The model under review builds one solid part; all positions refer to its coordinate system, in mm. Coordinates: 2 decimals unless noted, no trailing zeros. Order: outer loops, then holes, each group sorted by start corner. A loop starts at its lowest first (then second) coordinate and runs counter-clockwise, first axis right, second up. Notation, with made-up numbers: M 55,29 L 61,29 A23 cw 61,49 Z; hole C -3,19 d5. An arc over 180 degrees is marked long. Answer as CSV lines item,"result". Start each with the question number.
Q1. The part is to be moulded in two halves that separate along Z. For faces 1 (the face through (-3.45, -1.503, -19.963)), 2 (the face through (60.5, -2, -7)), 3 (the face through (45.473, -1.503, -11.382)), say which applies: +Z half, -Z half, draft (parallel to the pull), parting line (faces both ways), or undercut.
Q2. For P1, Ø6, axis at x = -46, z = 3, coming from the +Y side; P2, Ø1.5, axis at x = -42.5, y = -1.5, coming from the +Z side, all flat-tipped, find the tip position at first contact; note any pin that passes through.
Q3. Consider section A-A on x = -41. Write out the cut boundary in (y, z), and give its area (3 significant figures).
Q4. Consider section C-C on y = -0.8. Write out the cut boundary in (x, z).
Q5. Consider section D-D on x = -18. Write out the cut boundary in (y, z).
Q6. Wall thickness on L1, parallel to X at y = -0.15, z = -12; L2, parallel to X at y = -0.75, z = -11.5; L3, parallel to X at y = -2.5, z = 10.5: over which ranges is each line inside the solid? List them lowest first. Write a range as [from, to].
Q7. Consider section B-B on z = 5. Write out the cut boundary in (x, y).
from build123d import *

# Parameters (mm, degrees)
F0_R     = 2.7500072
F1_DEPTH = 3.048


# Not quite as in the source:
# - ends of sketch curves that miss each other by under 0.0002 mm in the source are joined


with BuildPart() as f1:
    # F0 (on Front) → F1 (new body)
    with BuildSketch(Plane.XZ):
        with BuildLine():
            ThreePointArc((60.500006, 12.486513), (59.7588291045, 13.4524362039), (58.6339869962, 12.986516621))
            Line((58.6339869962, 12.986516621), (57.9256398, 11.7596158))
            ThreePointArc((57.9256398, 11.7596158), (-4.481139989, -19.8585023044), (-58.5461372224, 24.5406923411))
            ThreePointArc((-58.5461372224, 24.5406923411), (-59.6518971954, 25.2287800004), (-60.4999806, 24.2403884))
            Line((-60.4999806, 24.2403884), (-60.4999806, -25.2403864))
            Line((-60.4999806, -25.2403864), (60.500006, -25.2403864))
            Line((60.500006, -25.2403864), (60.500006, 12.486513))
        make_face()
        with Locations((-42.4999912, -13.240385)):
            Circle(F0_R, mode=Mode.SUBTRACT)
        with Locations((47.5000066, -13.240385)):
            Circle(F0_R, mode=Mode.SUBTRACT)
    extrude(amount=F1_DEPTH)


solid = f1.part
Evaluation:
1,face 1,"+Z half"
1,face 2,"draft"
1,face 3,"undercut"
2,P1,"stops at y = 0"
2,P2,"stops at z = -0.99"
3,outline,"M -3.05,-25.24 L 0,-25.24 L 0,-15.55 L -3.05,-15.55 Z; M -3.05,-10.94 L 0,-10.94 L 0,-3.18 L -3.05,-3.18 Z"
3,area,"53.2 mm²"
4,outline,"M -60.5,-25.24 L 60.5,-25.24 L 60.5,12.49 A1 ccw 58.63,12.99 L 57.93,11.76 A64 cw -58.55,24.54 A1 ccw -60.5,24.24 Z; hole C -42.5,-13.24 d5.5; hole C 47.5,-13.24 d5.5"
5,outline,"M -3.05,-25.24 L 0,-25.24 L 0,-16.87 L -3.05,-16.87 Z"
6,L1,"x = [-60.5, -44.95], [-40.05, -28.91], [33.91, 45.05], [49.95, 60.5]"
6,L2,"x = [-60.5, -44.63], [-40.37, -29.79], [34.79, 45.37], [49.63, 60.5]"
6,L3,"x = [-60.5, -52.18], [57.18, 60.5]"
7,outline,"M -60.5,-3.05 L -48.43,-3.05 L -48.43,0 L -60.5,0 Z; M 53.43,-3.05 L 60.5,-3.05 L 60.5,0 L 53.43,0 Z"
